Could you check a few things on this model? Use its own coordinates, in mm. A direction names the side the tool comes from. Give positions to 0.01 mm unless a question says otherwise; leave off trailing zeros. Order: outer loops, then holes, each group sorted by start corner. A loop starts at its lowest first (then second) coordinate and runs counter-clockwise, first axis right, second up.
(1) If I drill on probe 1 along Y at (x, z) = (0, 4.25); probe 2 along Y at (x, z) = (0, 17); probe 3 along X at (y, z) = (-2, 8), over which ranges is the centre line in solid material (lowest first)?
(2) Imagine slicing it at D-D, the plane y = -8.75. Write out the boundary of the cut face in (x, z), then the cut area to 3 significant figures.
(3) Imagine slicing it at C-C, the plane z = 32.5. Write out the boundary of the cut face in (x, y).
(4) Will these pins go through, and if not, where does the flat tip stop? pin 1 (1 mm diameter, centred on y = 3, z = 8.5, fed in from -X); pin 2 (12 mm diameter, centred on x = -6, y = -10, fed in from +Z); pin 3 (3.5 mm diameter, centred on x = -0.5, y = -0.5, fed in from -Z).
(5) On a 3-axis mill with a long thin cutter (end or side, diameter ignored), from which of +Z, -Z, +X, -X, +Y, -Y can I reach the whole of each face in a straight line? I mean faces 4 (the flat face through (5.756, -9.785, 1.348)), 5 (the flat face through (5.25, 9.21, 3.57)), 6 (the cylindrical face through (0.023, -11.745, 3.629)), 7 (the flat face through (-5.25, -9.21, 3.57)). Say none if no direction works.
(6) Imagine slicing it at B-B, the plane z = 8.5. Write out the boundary of the cut face in (x, y).
(7) If we mould it in two halves opening along Y, with no side actions, what happens to faces 1 (the flat face through (5.17, 9.08, 5.85)), 2 (the flat face through (-10.6, 0, 4)), 3 (the flat face through (0, 0, 34))? For each: released by +Y, released by -Y, zero draft, split by the parting line, or undercut.
from build123d import *

# Parameters (mm, degrees)
BOSS_EXTRUDE1_DEPTH  = 1.5
SKETCH1_8_R          = 4.1
BOSS_EXTRUDE3_DEPTH  = 36
SKETCH1_9_R          = 5.05
BOSS_EXTRUDE4_DEPTH  = 19
SHELL1_START         = 2
SHELL1_OUTLINE_R     = 2.1
SHELL1_DEPTH         = 32
SHELL1_2_OUTLINE_R   = 3.05
SHELL1_2_OUTLINE_R_2 = 2.1
SHELL1_2_DEPTH       = 15
SKETCH1_10_R         = 3.25
CUT_EXTRUDE1_DEPTH   = 17
SKETCH1_3_R          = 3.25
BOSS_EXTRUDE2_DEPTH  = 6
CHAMFER1_SIZE        = 2
CHAMFER1_SIZE2       = 0.727940469
CHAMFER2_SIZE        = 2.747477419
CHAMFER2_SIZE_2      = 1
CHAMFER3_SIZE        = 1.212435565
CHAMFER3_SIZE_2      = 0.7
CHAMFER6_SIZE        = 0.3
FILLET1_R            = 3.2
CHAMFER5_SIZE        = 0.3
FILLET2_R            = 1
FILLET3_R            = 2


# Read off the part's stored shape, not the designer's step: Shell1
with BuildPart() as part:
    # Sketch1 → Boss-Extrude1 (new body)
    with BuildSketch(Plane.XY):
        Polygon((-11.5, 6.639528096), (0, 13.279056191), (11.5, 6.639528096), (11.5, -6.639528096), (0, -13.279056191), (-11.5, -6.639528096), align=None)
    extrude(amount=BOSS_EXTRUDE1_DEPTH)

    # Sketch1<8> → Boss-Extrude3 (add)
    with BuildSketch(Plane.XY):
        with Locations(Location((0, 0, 0), (0, 0, 180))):
            Circle(SKETCH1_8_R)
    extrude(amount=BOSS_EXTRUDE3_DEPTH)

    # Sketch1<9> → Boss-Extrude4 (add)
    with BuildSketch(Plane.XY):
        with Locations(Location((0, 0, 0), (0, 0, 180))):
            Circle(SKETCH1_9_R)
    extrude(amount=BOSS_EXTRUDE4_DEPTH)

    # Shell1 outline → Shell1 (cut)
    with BuildSketch(Plane.XY.offset(SHELL1_START)):
        Circle(SHELL1_OUTLINE_R)
    extrude(amount=SHELL1_DEPTH, mode=Mode.SUBTRACT)

    # Shell1 2 outline → Shell1 2 (cut)
    with BuildSketch(Plane.XY.offset(SHELL1_START)):
        Circle(SHELL1_2_OUTLINE_R)
        Circle(SHELL1_2_OUTLINE_R_2, mode=Mode.SUBTRACT)
    extrude(amount=SHELL1_2_DEPTH, mode=Mode.SUBTRACT)

    # Sketch1<10> → Cut-Extrude1 (cut)
    with BuildSketch(Plane.XY):
        Circle(SKETCH1_10_R)
    extrude(amount=CUT_EXTRUDE1_DEPTH, mode=Mode.SUBTRACT)

    # Sketch1<3> → Boss-Extrude2 (add)
    with BuildSketch(Plane.XY):
        Polygon((0, 12.239825707), (10.6, 6.119912853), (10.6, -6.119912853), (0, -12.239825707), (-10.6, -6.119912853), (-10.6, 6.119912853), align=None)
        Circle(SKETCH1_3_R, mode=Mode.SUBTRACT)
    extrude(amount=BOSS_EXTRUDE2_DEPTH)

    # Chamfer1
    chamfer1_edges = [part.edges().sort_by_distance(p)[0] for p in [
        (4.1, 0, 36),
    ]]
    chamfer1_side = [part.faces().sort_by_distance(p)[0] for p in [
        (4.1, 0, 27.5),
    ]]
    chamfer(chamfer1_edges, length=CHAMFER1_SIZE, length2=CHAMFER1_SIZE2, reference=chamfer1_side[0])

    # Chamfer2
    # the kernel refuses this chamfer: 2.747477419, 1 mm, written as the material it adds along each edge
    with BuildSketch(Plane(origin=(0, 0, 19), x_dir=(-1, 0, 0), z_dir=(0, -1, 0))) as chamfer2_piece_1_section:
        Polygon((4.1, -CHAMFER2_SIZE), (4.1 + CHAMFER2_SIZE_2, 0), (4.1, 0), align=None)
    chamfer2_piece_1 = revolve(axis=Axis((0, 0, 19), (0, 0, -1)), mode=Mode.PRIVATE)
    chamfer2_piece_1 = chamfer2_piece_1 & Plane(origin=(0, 0, 20.481947897), x_dir=(-1, 0, 0), z_dir=(0, 0, -1)) * Cylinder(5.05, 21, mode=Mode.PRIVATE)
    add(chamfer2_piece_1)

    # Chamfer3
    # the kernel refuses this chamfer: 1.212435565, 0.7 mm, written as the material it takes off along each edge
    with BuildSketch(Plane(origin=(0, 0, 17), x_dir=(1, 0, 0), z_dir=(0, -1, 0))) as chamfer3_piece_1_section:
        Polygon((2.1 + CHAMFER3_SIZE, 0), (2.1, CHAMFER3_SIZE_2), (2.1, 0), align=None)
    chamfer3_piece_1 = revolve(axis=Axis((0, 0, 17), (0, 0, 1)), mode=Mode.PRIVATE)
    chamfer3_piece_1 = chamfer3_piece_1 & Plane(origin=(0, 0, 17.363214185), x_dir=(1, 0, 0), z_dir=(0, 0, -1)) * Cylinder(3.25, 14, mode=Mode.PRIVATE)
    add(chamfer3_piece_1, mode=Mode.SUBTRACT)

    # Chamfer6
    chamfer6_edges = [part.edges().sort_by_distance(p)[0] for p in [
        (-3.25, 0, 0),
    ]]
    chamfer(chamfer6_edges, length=CHAMFER6_SIZE)

    # Fillet1
    fillet1_edges = [part.edges().sort_by_distance(p)[0] for p in [
        (-10.6, -6.119912853, 3.75),
        (0, -12.239825707, 3.75),
        (10.6, -6.119912853, 3.75),
        (10.6, 6.119912853, 3.75),
        (0, 12.239825707, 3.75),
        (-10.6, 6.119912853, 3.75),
    ]]
    fillet(fillet1_edges, radius=FILLET1_R)

    # Chamfer5
    chamfer5_edges = [part.edges().sort_by_distance(p)[0] for p in [
        (-5.3, -9.17986928, 6),
        (5.3, 9.17986928, 6),
        (-5.3, 9.17986928, 6),
        (-10.6, 0, 6),
        (10.171281292, 5.872391992, 6),
        (0, 11.744783984, 6),
        (-10.171281292, 5.872391992, 6),
        (-10.171281292, -5.872391992, 6),
        (0, -11.744783984, 6),
        (10.171281292, -5.872391992, 6),
        (5.75, 9.959292144, 1.5),
        (11.5, 0, 1.5),
        (5.75, -9.959292144, 1.5),
        (-5.75, -9.959292144, 1.5),
        (-11.5, 0, 1.5),
        (-5.75, 9.959292144, 1.5),
        (10.6, 0, 6),
        (5.3, -9.17986928, 6),
    ]]
    chamfer(chamfer5_edges, length=CHAMFER5_SIZE)

    # Fillet2
    fillet2_edges = [part.edges().sort_by_distance(p)[0] for p in [
        (11.5, 6.639528096, 0.6),
        (11.5, -6.639528096, 0.6),
        (0, -13.279056191, 0.6),
        (-11.5, -6.639528096, 0.6),
        (-11.5, 6.639528096, 0.6),
        (0, 13.279056191, 0.6),
    ]]
    fillet(fillet2_edges, radius=FILLET2_R)

    # Fillet3
    fillet3_edges = [part.edges().sort_by_distance(p)[0] for p in [
        (5.05, 0, 6),
    ]]
    fillet(fillet3_edges, radius=FILLET3_R)


solid = part.part
Answer block:
1. probe 1: y = -11.74 to -3.25, 3.25 to 11.74
1. probe 2: y = -5.05 to -3.25, 3.25 to 5.05
1. probe 3: x = -4.64 to -2.56, 2.56 to 4.64
2. outline: (-7.84, 0) - (7.84, 0) - (7.84, 1.2) - (7.24, 1.5) - (6.04, 1.5) - (6.04, 5.7) - (5.44, 6) - (-5.44, 6) - (-6.04, 5.7) - (-6.04, 1.5) - (-7.24, 1.5) - (-7.84, 1.2) - close
2. area: 77.6 mm2
3. outline: circle Ø8.2 at (0, 0); hole circle Ø4.2 at (0, 0)
4. pin 1: stops at x = -4.39
4. pin 2: stops at z = 6.56
4. pin 3: stops at z = 17.49
5. face 4: +Z, +X, -Y
5. face 5: +Z, +X, +Y
5. face 6: +Z, -Y
5. face 7: +Z, -X, -Y
6. outline: circle Ø10.1 at (0, 0); hole circle Ø6.5 at (0, 0)
7. face 1: released by +Y
7. face 2: zero draft
7. face 3: undercut
